```python
from build123d import *

# Parameters (mm, degrees)
SCHIZZO1_R                   = 3.5
ESTRUSIONE_ESTRUSIONE1_DEPTH = 5
SCHIZZO2_R                   = 2.5
ESTRUSIONE_ESTRUSIONE2_DEPTH = 24
SMUSSO1_SIZE                 = 0.25


with BuildPart() as part:
    # Schizzo1 → Estrusione-Estrusione1 (new body)
    with BuildSketch(Plane.XY):
        Circle(SCHIZZO1_R)
    extrude(amount=ESTRUSIONE_ESTRUSIONE1_DEPTH)

    # Schizzo2 → Estrusione-Estrusione2 (add)
    with BuildSketch(Plane.XY.offset(5)):
        Circle(SCHIZZO2_R)
    extrude(amount=ESTRUSIONE_ESTRUSIONE2_DEPTH)

    # Smusso1
    smusso1_edges = [part.edges().sort_by_distance(p)[0] for p in [
        (-3.5, 0, 0),
        (-3.5, 0, 5),
        (-2.5, 0, 29),
    ]]
    chamfer(smusso1_edges, length=SMUSSO1_SIZE)


solid = part.part
```
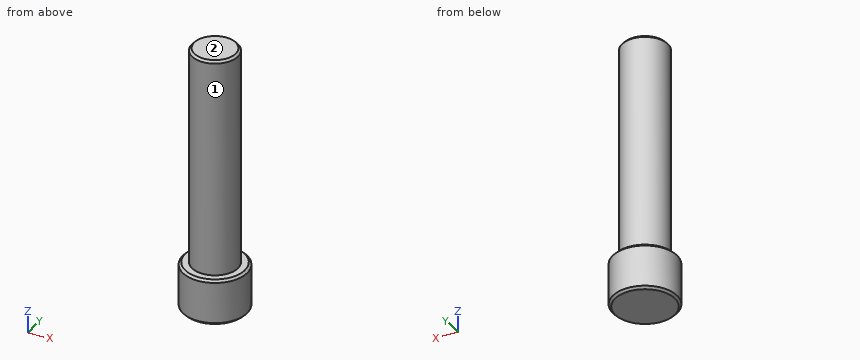
Check sheet for the modelled part. Datum: model origin and axes. Units: mm. Face numbers are marked on the shaded views. A direction names the side the tool comes from. Round coordinates to 2 decimals unless told otherwise and drop trailing zeros. Order: outer loops, then holes, each group sorted by start corner. A loop starts at its lowest first (then second) coordinate and runs counter-clockwise, first axis right, second up. Notation, with made-up numbers: (12.5, 47.5) - (51.5, 47.5) arc R27 ccw to (51.5, 77.5) - close; hole circle Ø4 at (40.5, 50). An arc over 180 degrees is marked (long way). Answer as CSV lines item,"result". Start each with the question number.
1) Tool access check on the marked faces 1 and 2. Record the directions out of +Z, -Z, +X, -X, +Y, -Y that give a thin tool (end or side, any length) a straight path to the whole face; none if there is none.
2) Section check C-C (z = 8.5). Record the cut outline in (x, y).
3) Section check A-A (x = 0). Record the cut outline in (y, z).
4) Depth check by flat-ended pin: pin 1 (3 mm diameter, centred on y = -1, z = 14.5, fed in from +X); pin 2 (4 mm diameter, centred on x = -0.5, z = 15.5, fed in from +Y); pin 3 (2 mm diameter, centred on x = 2.5, z = 8, fed in from +Y). Enter the tip coordinate at first touch or a pass-through.
5) Scan lines: probe 1 along Z at (x, y) = (-2, -2.25); probe 2 along Y at (x, z) = (0, 23.5); probe 3 along Z at (x, y) = (-1.75, -3). Record each from-to range of solid material in increasing order.
Determined:
1,face 1,"+Z"
1,face 2,"+Z, +X, -X, +Y, -Y"
2,outline,"circle Ø5 at (0, 0)"
3,outline,"(-3.5, 0.25) - (-3.25, 0) - (3.25, 0) - (3.5, 0.25) - (3.5, 4.75) - (3.25, 5) - (2.5, 5) - (2.5, 28.75) - (2.25, 29) - (-2.25, 29) - (-2.5, 28.75) - (-2.5, 5) - (-3.25, 5) - (-3.5, 4.75) - close"
4,pin 1,"x = 2.5"
4,pin 2,"y = 2.5"
4,pin 3,"y = 2"
5,probe 1,"0 to 5"
5,probe 2,"-2.5 to 2.5"
5,probe 3,"0.22 to 4.78"
